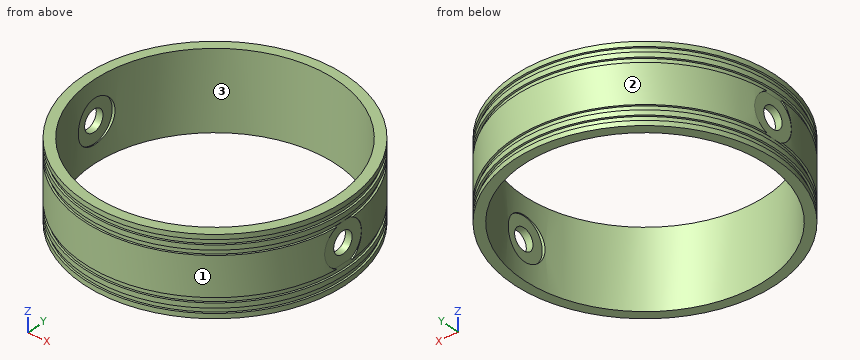
```python
from build123d import *

# Parameters (mm, degrees)
SKETCH005_R      = 140.350312
SKETCH005_R_2    = 133
EXTRUDE011_DEPTH = 5
EXTRUDE010_DEPTH = 5
EXTRUDE008_DEPTH = 5
EXTRUDE009_DEPTH = 5
SKETCH004_R      = 157.293563
EXTRUDE007_DEPTH = 50
SKETCH003_R      = 22
EXTRUDE004_DEPTH = 10
EXTRUDE005_DEPTH = 10
EXTRUDE006_DEPTH = 10
EXTRUDE002_DEPTH = 10
SKETCH002_R      = 11
EXTRUDE_DEPTH    = 150
SKETCH_R         = 134.952227
SKETCH_R_2       = 125
EXTRUDE001_DEPTH = 80


with BuildPart() as extrude011:
    # Sketch005 → Extrude011 (new body)
    with BuildSketch(Plane.XY):
        Circle(SKETCH005_R)
        Circle(SKETCH005_R_2, mode=Mode.SUBTRACT)
    extrude(amount=EXTRUDE011_DEPTH)


with BuildPart() as extrude011_1:
    # Extrude011 placement: moved
    add(extrude011.part.moved(Location((0, 0, -35))))


with BuildPart() as extrude010:
    # Sketch005 → Extrude010 (new body)
    with BuildSketch(Plane.XY):
        Circle(SKETCH005_R)
        Circle(SKETCH005_R_2, mode=Mode.SUBTRACT)
    extrude(amount=EXTRUDE010_DEPTH)


with BuildPart() as extrude010_1:
    # Extrude010 placement: moved
    add(extrude010.part.moved(Location((0, 0, -25))))


with BuildPart() as extrude008:
    # Sketch005 → Extrude008 (new body)
    with BuildSketch(Plane.XY):
        Circle(SKETCH005_R)
        Circle(SKETCH005_R_2, mode=Mode.SUBTRACT)
    extrude(amount=EXTRUDE008_DEPTH)


with BuildPart() as extrude008_1:
    # Extrude008 placement: moved
    add(extrude008.part.moved(Location((0, 0, 20))))


with BuildPart() as extrude009:
    # Sketch005 → Extrude009 (new body)
    with BuildSketch(Plane.XY):
        Circle(SKETCH005_R)
        Circle(SKETCH005_R_2, mode=Mode.SUBTRACT)
    extrude(amount=EXTRUDE009_DEPTH)


with BuildPart() as extrude009_1:
    # Extrude009 placement: moved
    add(extrude009.part.moved(Location((0, 0, 30))))


with BuildPart() as extrude007:
    # Sketch004 → Extrude007 (new body)
    with BuildSketch(Plane.XY):
        Circle(SKETCH004_R)
    extrude(amount=EXTRUDE007_DEPTH)


with BuildPart() as extrude007_1:
    # Extrude007 placement: moved
    add(extrude007.part.moved(Location((0, 0, 51))))


with BuildPart() as extrude004:
    # Sketch003 (on Face3 of Extrude) → Extrude004 (new body)
    with BuildSketch(Plane.YZ.offset(150)):
        Circle(SKETCH003_R)
    extrude(amount=-EXTRUDE004_DEPTH)


with BuildPart() as extrude004_1:
    # Extrude004 placement: moved
    add(extrude004.part.moved(Location((-283, 0, 0))))


with BuildPart() as extrude005:
    # Sketch003 (on Face3 of Extrude) → Extrude005 (new body)
    with BuildSketch(Plane.YZ.offset(150)):
        Circle(SKETCH003_R)
    extrude(amount=-EXTRUDE005_DEPTH)


with BuildPart() as extrude005_1:
    # Extrude005 placement: moved
    add(extrude005.part.moved(Location((-266, 0, 0))))


with BuildPart() as extrude006:
    # Sketch003 (on Face3 of Extrude) → Extrude006 (new body)
    with BuildSketch(Plane.YZ.offset(150)):
        Circle(SKETCH003_R)
    extrude(amount=-EXTRUDE006_DEPTH)


with BuildPart() as extrude006_1:
    # Extrude006 placement: moved
    add(extrude006.part.moved(Location((-24, 0, 0))))


with BuildPart() as extrude002:
    # Sketch003 (on Face3 of Extrude) → Extrude002 (new body)
    with BuildSketch(Plane.YZ.offset(150)):
        Circle(SKETCH003_R)
    extrude(amount=-EXTRUDE002_DEPTH)


with BuildPart() as extrude002_1:
    # Extrude002 placement: moved
    add(extrude002.part.moved(Location((-7, 0, 0))))


with BuildPart() as extrude_body:
    # Sketch002 → Extrude (new body, symmetric)
    with BuildSketch(Plane.YZ):
        Circle(SKETCH002_R)
    extrude(amount=EXTRUDE_DEPTH, both=True)


with BuildPart() as cut009:
    # Sketch → Extrude001 (new body)
    with BuildSketch(Plane.XY):
        Circle(SKETCH_R)
        Circle(SKETCH_R_2, mode=Mode.SUBTRACT)
    extrude(amount=EXTRUDE001_DEPTH)


with BuildPart() as cut009_1:
    # Extrude001 placement: moved
    add(cut009.part.moved(Location((0, 0, -40))))

    # Cut: cut Extrude body
    add(extrude_body.part, mode=Mode.SUBTRACT)

    # Cut001: cut Extrude002
    add(extrude002_1.part, mode=Mode.SUBTRACT)

    # Cut002: cut Extrude006
    add(extrude006_1.part, mode=Mode.SUBTRACT)

    # Cut003: cut Extrude005
    add(extrude005_1.part, mode=Mode.SUBTRACT)

    # Cut004: cut Extrude004
    add(extrude004_1.part, mode=Mode.SUBTRACT)

    # Cut005: cut Extrude007
    add(extrude007_1.part, mode=Mode.SUBTRACT)

    # Cut006: cut Extrude009
    add(extrude009_1.part, mode=Mode.SUBTRACT)

    # Cut007: cut Extrude008
    add(extrude008_1.part, mode=Mode.SUBTRACT)

    # Cut008: cut Extrude010
    add(extrude010_1.part, mode=Mode.SUBTRACT)

    # Cut009: cut Extrude011
    add(extrude011_1.part, mode=Mode.SUBTRACT)


solid = cut009_1.part
```
For this review, take the finished solid that the model builds, in its own axes (mm). Face numbers are marked on the shaded views. Round coordinates to 2 decimals unless told otherwise and drop trailing zeros. Order: outer loops, then holes, each group sorted by start corner. A loop starts at its lowest first (then second) coordinate and runs counter-clockwise, first axis right, second up.
Q1. We need section A-A, the plane z = -6.5. Give the boundary of the cut face in (x, y), plus the area to 3 significant figures.
Findings below:
outline: (-133.31, -21.02) arc R134.95 ccw to (133.31, -21.02) - (133, -21.02) - (133, -8.87) - (126, -8.87) - (126, -21.02) - (123.22, -21.02) arc R125 cw to (-123.22, -21.02) - (-126, -21.02) - (-126, -8.87) - (-133, -8.87) - (-133, -21.02) - close; (-133.31, 21.02) - (-133, 21.02) - (-133, 8.87) - (-126, 8.87) - (-126, 21.02) - (-123.22, 21.02) arc R125 cw to (123.22, 21.02) - (126, 21.02) - (126, 8.87) - (133, 8.87) - (133, 21.02) - (133.31, 21.02) arc R134.95 ccw to start
area: 7,630 mm2
Q2. Wall thickness on line 1 (X direction, y = 0, z = 18); line 2 (Z direction, x = 129.25, y = 0); line 3 (Y direction, x = 0, z = 34): over which ranges is each line inside the solid? List them lowest first.
Findings below:
line 1: x = -133 to -126, 126 to 133
line 2: z = -40 to -11, 11 to 40
line 3: y = -133 to -125, 125 to 133
Q3. Insertion check: P1, Ø2, axis at x = 51.5, z = 10, coming from the +Y side; P2, Ø3, axis at y = -64, z = -6.5, coming from the +X side; P3, Ø6, axis at y = 89, z = -3.5, coming from the -X side. Each pin has a flat end and moves straight along its axis. Give the tip position at first contact, or say it passes through.
Findings below:
P1: stops at y = 125.15
P2: stops at x = 119.61
P3: stops at x = -104
Q4. We need section B-B, the plane z = 15. Give the boundary of the cut face in (x, y).
Findings below:
outline: (-133.99, -16.09) arc R134.95 ccw to (133.99, -16.09) - (133, -16.09) - (133, 16.09) - (133.99, 16.09) arc R134.95 ccw to (-133.99, 16.09) - (-133, 16.09) - (-133, -16.09) - close; hole (-126, -16.09) - (-123.96, -16.09) arc R125 ccw to (123.96, -16.09) - (126, -16.09) - (126, 16.09) - (123.96, 16.09) arc R125 ccw to (-123.96, 16.09) - (-126, 16.09) - close
Q5. Mouldability with a two-part tool opening along Y and no side actions: class the marked faces 1, 2 and 3 as pulls with the +Y half, pulls with the -Y half, needs draft (parallel to the pull), parting line crosses it, or undercut.
Findings below:
face 1: pulls with the -Y half
face 2: pulls with the +Y half
face 3: undercut
